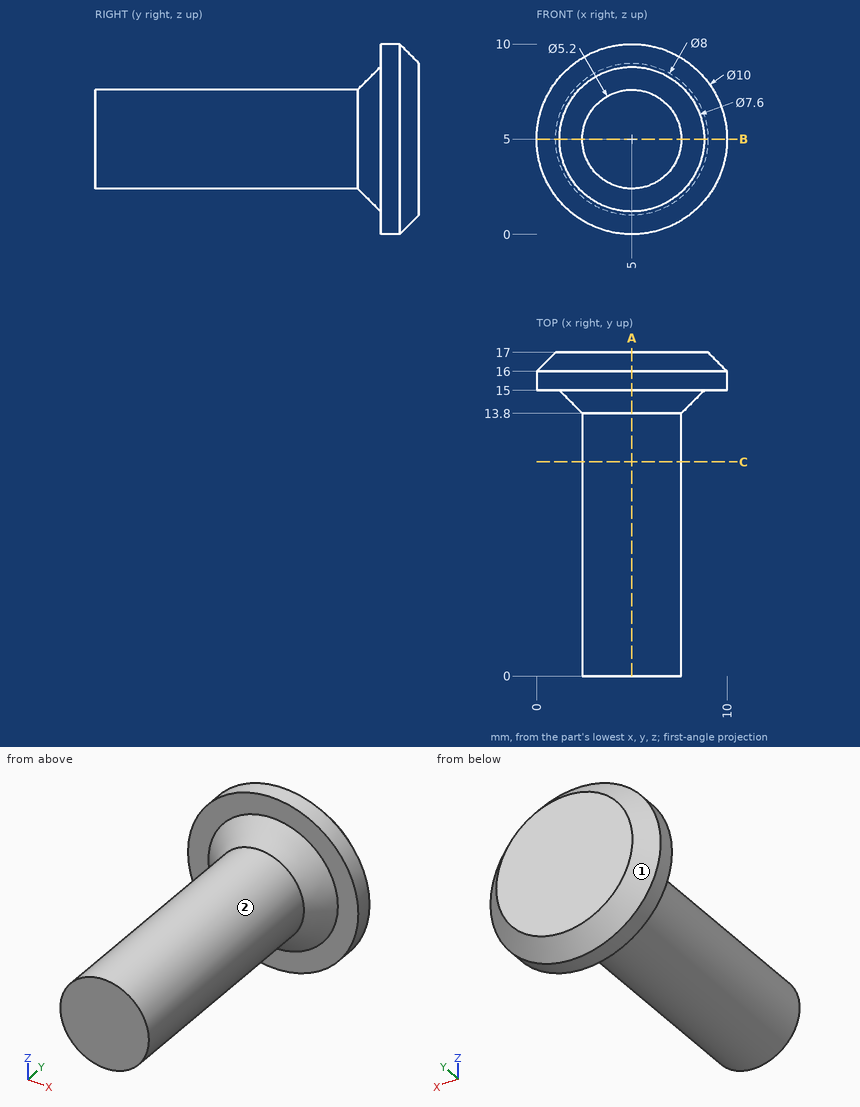
The figure shows three views and two pictorial views of one solid part (mm, origin at its lowest corner). Answer the questions. A direction names the side the tool comes from. Round coordinates to 2 decimals unless told otherwise and drop trailing zeros. Write each loop counter-clockwise with the first axis right and the second up, starting at its lowest first coordinate (ties: lowest second). Pieces come first, ordered by that corner, then holes. Notation, with made-up numbers: M 17,50.25 L 64,50.25 A17 cw 64,66.25 Z; hole C 47,30 d1. An arc over 180 degrees is marked long. Use a Markdown table: item, result.
1) Consider line 1 (X direction, y = 8.75, z = 5); line 2 (X direction, y = 14, z = 7.5); line 3 (Z direction, x = 2.75, y = 15.75). Determine where each line is inside the solid, lowest interval first. Write a range as [from, to].
Taken from the geometry:
| item | result |
|---|---|
| line 1 | x = [2.4, 7.6] |
| line 2 | x = [3.74, 6.26] |
| line 3 | z = [0.53, 9.47] |
2) The part is cut by section C-C on y = 11.25. Give the vertices of the cut face in (x, z), plus the area to 3 significant figures.
Taken from the geometry:
| item | result |
|---|---|
| outline | C 5,5 d5.2 |
| area | 21.2 mm2 |
3) Flat-ended cylindrical pins translate along their axes: pin 1 (1 mm diameter, centred on x = 2.5, y = 12, fed in from -Z); pin 2 (4 mm diameter, centred on x = 8.5, z = 1, fed in from +Y); pin 3 (3 mm diameter, centred on y = 5, z = 5.5, fed in from +X); pin 4 (2 mm diameter, centred on y = 7.5, z = 2.5, fed in from +X). Find the tip coordinate at first contact, or state that the pin passes through.
Taken from the geometry:
| item | result |
|---|---|
| pin 1 | stops at z = 3.34 |
| pin 2 | stops at y = 17 |
| pin 3 | stops at x = 7.6 |
| pin 4 | stops at x = 7.12 |
4) The part is cut by section B-B on z = 5. Give the vertices of the cut face in (x, y).
Taken from the geometry:
| item | result |
|---|---|
| outline | M 0,15 L 1.2,15 L 2.4,13.8 L 2.4,0 L 7.6,0 L 7.6,13.8 L 8.8,15 L 10,15 L 10,16 L 9,17 L 1,17 L 0,16 Z |
5) The part is cut by section A-A on x = 5. Give the vertices of the cut face in (y, z).
Taken from the geometry:
| item | result |
|---|---|
| outline | M 0,2.4 L 13.8,2.4 L 15,1.2 L 15,0 L 16,0 L 17,1 L 17,9 L 16,10 L 15,10 L 15,8.8 L 13.8,7.6 L 0,7.6 Z |
6) Which of the six approach directions +Z, -Z, +X, -X, +Y, -Y give full straight-line access (tool end or side, diameter ignored) to the marked faces 1 and 2?
Taken from the geometry:
| item | result |
|---|---|
| face 1 | +Y |
| face 2 | -Y |
